```python
from build123d import *

# Parameters (mm, degrees)
SKETCH_1_R               = 1.25
EXTRUDE_3_DEPTH          = 3
SKETCH_2_W               = 18
SKETCH_2_H               = 18
EXTRUDE_4_DEPTH          = 17
SKETCH_3_R               = 0.85
CUT_EXTRUDE_2_DEPTH      = 12
SKETCH_4_R               = 0.75
CUT_EXTRUDE_4_DEPTH      = 18
SKETCH_5_R               = 0.75
CUT_EXTRUDE_5_DEPTH      = 18
SKETCH_6_R               = 1.5
SKETCH_6_R_2             = 0.75
EXTRUDE_7_DEPTH          = 8
SKETCH_10_R              = 1.25
SKETCH_10_R_2            = 0.85
EXTRUDE_13_DEPTH         = 8
PATTERN_CIRCULAR_1_COUNT = 4


with BuildPart() as part:
    # 草图1 → 凸台-拉伸3 (new body)
    with BuildSketch(Plane.XY):
        with BuildLine():
            Line((-11, -18), (11, -18))
            ThreePointArc((11, -18), (15.949747468, -15.949747468), (18, -11))
            Line((18, -11), (18, 11))
            ThreePointArc((18, 11), (15.949747468, 15.949747468), (11, 18))
            Line((11, 18), (-11, 18))
            ThreePointArc((-11, 18), (-15.949747468, 15.949747468), (-18, 11))
            Line((-18, 11), (-18, -11))
            ThreePointArc((-18, -11), (-15.949747468, -15.949747468), (-11, -18))
        make_face()
        with Locations((13, 13)):
            Circle(SKETCH_1_R, mode=Mode.SUBTRACT)
        with Locations((-13, 13)):
            Circle(SKETCH_1_R, mode=Mode.SUBTRACT)
        with Locations((-13, -13)):
            Circle(SKETCH_1_R, mode=Mode.SUBTRACT)
        with Locations((13, -13)):
            Circle(SKETCH_1_R, mode=Mode.SUBTRACT)
    extrude(amount=EXTRUDE_3_DEPTH)

    # 草图2 → 凸台-拉伸4 (add)
    with BuildSketch(Plane.XY):
        Rectangle(SKETCH_2_W, SKETCH_2_H)
    extrude(amount=-EXTRUDE_4_DEPTH)

    # 草图3 → 切除-拉伸2 (cut)
    with BuildSketch(Plane(origin=(0, 0, -17), x_dir=(-1, 0, 0), z_dir=(0, 0, -1))):
        Circle(SKETCH_3_R)
    extrude(amount=-CUT_EXTRUDE_2_DEPTH, mode=Mode.SUBTRACT)

    # 草图4 → 切除-拉伸4 (cut)
    with BuildSketch(Plane.ZY.offset(9)):
        with Locations((-7, 0)):
            Circle(SKETCH_4_R)
    extrude(amount=-CUT_EXTRUDE_4_DEPTH, mode=Mode.SUBTRACT)

    # 草图5 → 切除-拉伸5 (cut)
    with BuildSketch(Plane(origin=(0, 9, 0), x_dir=(1, 0, 0), z_dir=(0, 1, 0))):
        with Locations((0, 7)):
            Circle(SKETCH_5_R)
    extrude(amount=-CUT_EXTRUDE_5_DEPTH, mode=Mode.SUBTRACT)

    # 草图6 → 凸台-拉伸7 (add)
    with BuildSketch(Plane.ZY.offset(9)):
        with Locations((-7, 0)):
            Circle(SKETCH_6_R)
        with Locations((-7, 0)):
            Circle(SKETCH_6_R_2, mode=Mode.SUBTRACT)
    extrude_7 = extrude(amount=EXTRUDE_7_DEPTH)

    # 草图10 → 凸台-拉伸13 (add)
    with BuildSketch(Plane(origin=(0, 0, -17), x_dir=(-1, 0, 0), z_dir=(0, 0, -1))):
        Circle(SKETCH_10_R)
        Circle(SKETCH_10_R_2, mode=Mode.SUBTRACT)
    extrude(amount=EXTRUDE_13_DEPTH)

    # 阵列(圆周)1: 凸台-拉伸7 ×4 about axis
    pattern_circular_1_axis = Axis((0, 0, 0), (0, 0, 1))
    for i in range(1, PATTERN_CIRCULAR_1_COUNT):
        add(extrude_7.rotate(pattern_circular_1_axis, i * 360 / PATTERN_CIRCULAR_1_COUNT))


solid = part.part
```
Check sheet for the modelled part. Datum: model origin and axes. Units: mm. A direction names the side the tool comes from. Coordinates: 2 decimals unless noted, no trailing zeros. Loops run counter-clockwise (first coordinate to the right, second up) from the corner with the lowest first, then second, coordinate; pieces in that order, holes last. Notation, with made-up numbers: M -31.5,9 L 2.5,9 A21 cw 2.5,37 Z; hole C -27.75,-26.75 d11. An arc over 180 degrees is marked long. Answer as a JSON object with one key per item and string values.
1. Sectioned sample at B-B on x = 13. Record the cut outline in (y, z), and give its area (3 significant figures).
Outcome:
{"outline": "M -17.71,0 L -14.25,0 L -14.25,3 L -17.71,3 Z; M -11.75,0 L 11.75,0 L 11.75,3 L -11.75,3 Z; C 0,-7 d3; M 14.25,0 L 17.71,0 L 17.71,3 L 14.25,3 Z; hole C 0,-7 d1.5", "area": "96.6 mm²"}
2. Scan lines: L1, parallel to Z at x = 0, y = -11.25; L2, parallel to Y at x = 10.75, z = -7; L3, parallel to Y at x = -5, z = -7. Record each from-to range of solid material in increasing order. Write a range as from..to.
Outcome:
{"L1": "-8.5..-7.75, -6.25..-5.5, 0..3", "L2": "-1.5..-0.75, 0.75..1.5", "L3": "-9..-0.75, 0.75..9"}
3. Release check for a two-part mould opening along Z. For faces 5 (the cylindrical face through (8.69, -0.03, -7.75)), 6 (the flat face through (0, 0, -5)), 7 (the cylindrical face through (-13.921, -12.155, 1.479)) record: pulls with the +Z half, pulls with the -Z half, needs draft (parallel to the pull), parting line crosses it, or undercut.
Outcome:
{"face 5": "undercut", "face 6": "pulls with the -Z half", "face 7": "needs draft"}
4. Access from +Z, -Z, +X, -X, +Y, -Y to the whole of each face (thin tool, end or side, straight path). Record for faces 1 (the cylindrical face through (0.07, 12.94, -8.5)), 2 (the flat face through (17, -1, -7)), 3 (the flat face through (0, -12, 0)), 4 (the flat face through (-17, 1, -7)).
Outcome:
{"face 1": "+Y", "face 2": "-Z, +X, +Y, -Y", "face 3": "none", "face 4": "-Z, -X, +Y, -Y"}
5. Sectioned sample at C-C on y = -12.5. Record the cut outline in (x, z), and give its area (3 significant figures).
Outcome:
{"outline": "M -17.84,0 L -14.15,0 L -14.15,3 L -17.84,3 Z; M -11.85,0 L 11.85,0 L 11.85,3 L -11.85,3 Z; C 0,-7 d3; M 14.15,0 L 17.84,0 L 17.84,3 L 14.15,3 Z; hole C 0,-7 d1.5", "area": "98.6 mm²"}
6. Sectioned sample at A-A on y = 0. Count the separate pieces of the cut face and the enclosed holes in it, and give its area (3 significant figures).
Outcome:
{"separate pieces": "3", "enclosed holes": "0", "area": "400 mm²"}
7. Sectioned sample at D-D on z = -15. Record the cut outline in (x, y), and give its area (3 significant figures).
Outcome:
{"outline": "M -9,-9 L 9,-9 L 9,9 L -9,9 Z; hole C 0,0 d1.7", "area": "322 mm²"}
8. Depth check by flat-ended pin: P1, Ø1.7, axis at x = 0, z = -7, coming from the +Y side; P2, Ø5.5, axis at x = -3.5, y = -2, coming from the -Z side; P3, Ø3, axis at x = 13, y = 13, coming from the -Z side. Enter the tip coordinate at first touch or a pass-through.
Outcome:
{"P1": "y = 17", "P2": "z = -17", "P3": "z = 0"}
